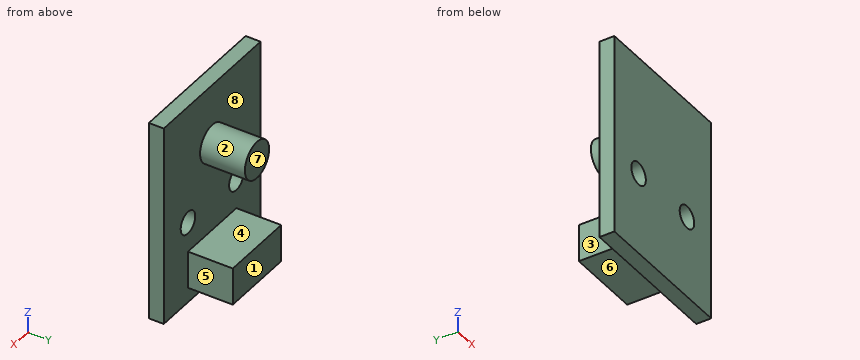
Autodesk Inventor part; units mm, degrees
ref_plane "YZ Plane" through (0, 0, 0) normal (1, 0, 0) x (0, 1, 0)
ref_plane "XZ Plane" through (0, 0, 0) normal (0, 1, 0) x (-1, 0, 0)
ref_plane "XY Plane" through (0, 0, 0) normal (0, 0, 1) x (1, 0, 0)
sketch "스케치1" plane through (0, 0, 0) normal (0, 1, 0) x (-1, 0, 0)
  line L0 (0, 0) -> (-20, 0)
  line L1 (-20, 0) -> (-20, -27)
  line L2 (-20, -27) -> (0, -27)
  line L3 (0, -27) -> (0, 0)
  dimension "d0" = 20
  dimension "d1" = 27
extrude "돌출1" add sketch "스케치1" along normal blind 2
sketch "스케치2" plane through (0, 2, 0) normal (0, 1, 0) x (1, 0, 0)
  line L0 (0, 0) -> (20, 0)
  line L1 (20, 0) -> (20, 27)
  line L2 (20, 27) -> (0, 27)
  line L3 (0, 27) -> (0, 0)
  line L4 (5, 20) -> (15, 20)
  line L5 (15, 20) -> (15, 25)
  line L6 (15, 25) -> (5, 25)
  line L7 (5, 25) -> (5, 20)
  dimension "d4" = 5
  dimension "d5" = 2
  dimension "d6" = 5
  dimension "d7" = 10
extrude "돌출2" add sketch "스케치2" along normal blind 6 contours L7 L6 L5 L4
sketch "스케치3" plane through (0, 2, 0) normal (0, 1, 0) x (1, 0, 0)
  line L0 (5, 20) -> (5, 25)
  line L1 (5, 25) -> (15, 25)
  line L2 (15, 25) -> (15, 20)
  line L3 (15, 20) -> (5, 20)
  line L4 (0, 0) -> (20, 0)
  line L5 (20, 0) -> (20, 27)
  line L6 (20, 27) -> (0, 27)
  line L7 (0, 27) -> (0, 0)
  circle A0 centre (10, 8) radius 2.5
  dimension "d10" = 5
  dimension "d11" = 8
extrude "돌출3" add sketch "스케치3" along normal blind 6 contours A0
sketch "스케치4" plane through (0, 2, 0) normal (0, 1, 0) x (1, 0, 0)
  circle A0 centre (10, 8) radius 2.5
  line L0 (5, 20) -> (5, 25)
  line L1 (5, 25) -> (15, 25)
  line L2 (15, 25) -> (15, 20)
  line L3 (15, 20) -> (5, 20)
  line L4 (0, 0) -> (20, 0)
  line L5 (20, 0) -> (20, 27)
  line L6 (20, 27) -> (0, 27)
  line L7 (0, 27) -> (0, 0)
  circle A1 centre (5, 16) radius 1.5
  circle A2 centre (15, 16) radius 1.5
  dimension "d14" = 3
  dimension "d15" = 3
  dimension "d16" = 5
  dimension "d17" = 11
  dimension "d18" = 11
  dimension "d19" = 5
extrude "돌출4" cut sketch "스케치4" against normal blind 6 contours A1 | A2
properties part number "CdS모듈"
The listing builds one solid part. Answer for the finished solid, in the listing's coordinates (mm). Face numbers are marked on the shaded views. A direction names the side the tool comes from. Coordinates: 2 decimals unless noted, no trailing zeros. Write each loop counter-clockwise with the first axis right and the second up, starting at its lowest first coordinate (ties: lowest second). Pieces come first, ordered by that corner, then holes. Notation, with made-up numbers: M -11.75,60 L -4.75,60 A10 cw -4.75,69 Z; hole C -23.5,88 d8. An arc over 180 degrees is marked long. Use a Markdown table: item, result. Add a question column.
1. Section A-A (z = -16) is taken. Give the vertices of the cut face in (x, y), plus the area to 3 significant figures.
2. Given P1, Ø3.5, axis at x = 5, z = -16, coming from the +Y side; P2, Ø1.5, axis at x = 11.5, y = 7, coming from the +Z side; P3, Ø2.5, axis at x = 15, z = -16, coming from the +Y side; P4, Ø6, axis at x = 12, z = -6, coming from the +Y side, each flat-ended and moving along its own axis, determine where each tip first touches the part or whether it passes through.
3. Section D-D (y = 5.75) is taken. Give the vertices of the cut face in (x, z).
4. Straight lines are drawn through the part: line 1 along X through (y, z) = (0.7, -16); line 2 along Z through (x, y) = (15, 0.55); line 3 along Y through (x, z) = (14, -3.25). For each, find the intervals that lie inside material, in ascending order. Write a range as [from, to].
5. Section C-C (z = -8) is taken. Give the vertices of the cut face in (x, y).
6. Which of the six approach directions +Z, -Z, +X, -X, +Y, -Y give full straight-line access (tool end or side, diameter ignored) to the marked faces 1, 2, 3, 4 and 5?
7. For a pull along Z with two mould halves and no side action, classify the marked faces 6, 7 and 8 as +Z half, -Z half, draft (parallel to the pull), parting line (faces both ways), or undercut.
8. Section B-B (x = 4) is taken. Give the vertices of the cut face in (y, z), plus the area to 3 significant figures.
Data:
| question | item | result |
|---|---|---|
| 1 | outline | M 0,0 L 3.5,0 L 3.5,2 L 0,2 Z; M 6.5,0 L 13.5,0 L 13.5,2 L 6.5,2 Z; M 16.5,0 L 20,0 L 20,2 L 16.5,2 Z |
| 1 | area | 28.0 mm2 |
| 2 | P1 | stops at y = 2 |
| 2 | P2 | stops at z = -5.62 |
| 2 | P3 | passes through |
| 2 | P4 | stops at y = 8 |
| 3 | outline | M 5,-25 L 15,-25 L 15,-20 L 5,-20 Z; C 10,-8 d5 |
| 4 | line 1 | x = [0, 3.5], [6.5, 13.5], [16.5, 20] |
| 4 | line 2 | z = [-27, -17.5], [-14.5, 0] |
| 4 | line 3 | y = [0, 2] |
| 5 | outline | M 0,0 L 20,0 L 20,2 L 12.5,2 L 12.5,8 L 7.5,8 L 7.5,2 L 0,2 Z |
| 6 | face 1 | +Z, -Z, +X, -X, +Y |
| 6 | face 2 | +Y |
| 6 | face 3 | +Z, -Z, -X, +Y |
| 6 | face 4 | +X, -X, +Y |
| 6 | face 5 | +Z, -Z, +X, +Y |
| 7 | face 6 | -Z half |
| 7 | face 7 | draft |
| 7 | face 8 | undercut |
| 8 | outline | M 0,-27 L 2,-27 L 2,-17.12 L 0,-17.12 Z; M 0,-14.88 L 2,-14.88 L 2,0 L 0,0 Z |
| 8 | area | 49.5 mm2 |
